Input: dimensioned drawing with shaded views. Units: mm. Origin: part minimum x, y, z. A direction names the side the tool comes from. Round coordinates to 2 decimals unless told otherwise and drop trailing zeros. Loops run counter-clockwise (first coordinate to the right, second up) from the corner with the lowest first, then second, coordinate; pieces in that order, holes last. Notation, with made-up numbers: M -12.75,-12 L 14.25,-12 A21 ccw 14.25,4 Z; hole C 70.5,4.25 d10. An arc over 180 degrees is marked long. Answer as a JSON object with one key per item and string values.
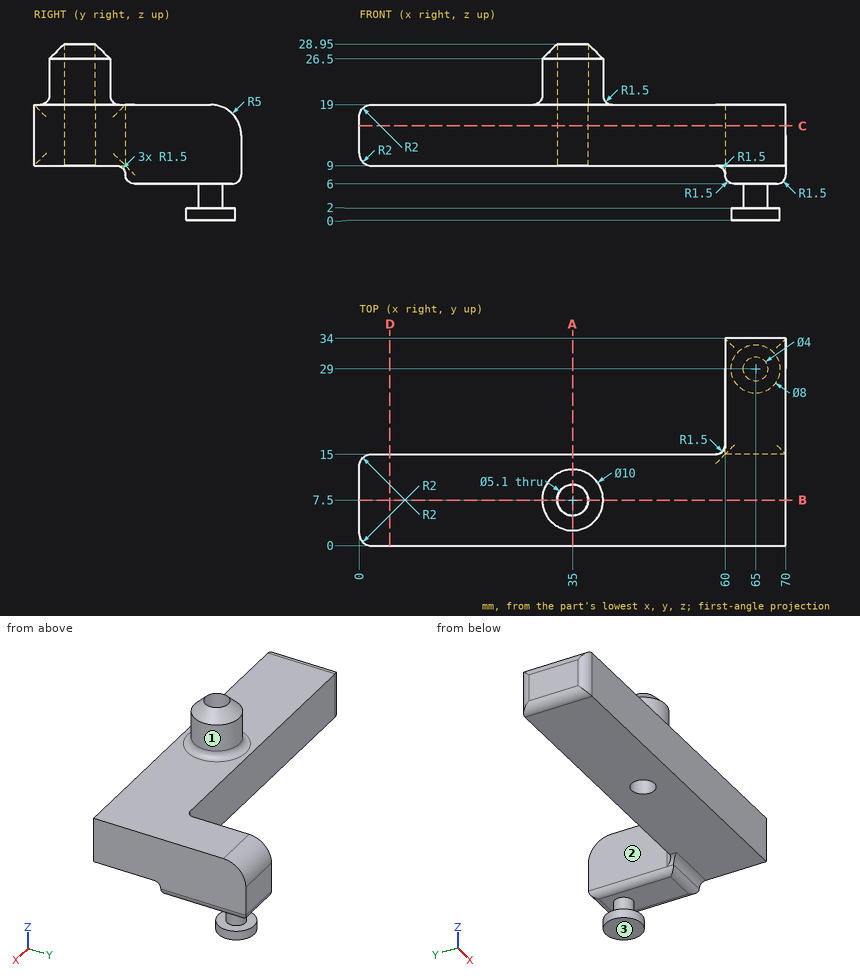
Item 1: Section B-B on y = 7.5. Return the cut outline in (x, z).
Answer sheet:
{"outline": "M 0,11 A2 ccw 2,9 L 32.45,9 L 32.45,28.95 L 30,26.5 L 30,20.5 A1.5 cw 28.5,19 L 2,19 A2 ccw 0,17 Z; M 37.55,9 L 70,9 L 70,19 L 41.5,19 A1.5 cw 40,20.5 L 40,26.5 L 37.55,28.95 Z"}
Item 2: Section C-C on z = 15.5. Return the cut outline in (x, y).
Answer sheet:
{"outline": "M 0,2 A2 ccw 2,0 L 70,0 L 70,33.77 L 60,33.77 L 60,16.5 A1.5 cw 58.5,15 L 2,15 A2 ccw 0,13 Z; hole C 35,7.5 d5.1"}
Item 3: Access query for the marked faces 1, 2 and 3. Directions: +Z, -Z, +X, -X, +Y, -Y. A direction counts if a zero-diameter tool reaches every point of the face in a straight line with its end or side. Return the directions, or none.
Answer sheet:
{"face 1": "+Z", "face 2": "+Z, -Z, -X, +Y", "face 3": "-Z, +X, -X, +Y, -Y"}
Item 4: Section A-A on x = 35. Return the cut outline in (y, z).
Answer sheet:
{"outline": "M 0,9 L 4.95,9 L 4.95,28.95 L 2.5,26.5 L 2.5,20.5 A1.5 cw 1,19 L 0,19 Z; M 10.05,9 L 15,9 L 15,19 L 14,19 A1.5 cw 12.5,20.5 L 12.5,26.5 L 10.05,28.95 Z"}
Item 5: Line query: probe 1 along Y at (x, z) = (35, 16); probe 2 along Y at (x, z) = (35, 24.25); probe 3 along X at (y, z) = (21, 13). Output: solid intervals per line, ascending. Write a range as from..to.
Answer sheet:
{"probe 1": "y = 0..4.95, 10.05..15", "probe 2": "y = 2.5..4.95, 10.05..12.5", "probe 3": "x = 60..70"}
Item 6: Section D-D on x = 5. Return the cut outline in (y, z), then the cut area to 3 significant figures.
Answer sheet:
{"outline": "M 0,9 L 15,9 L 15,19 L 0,19 Z", "area": "150 mm²"}
Item 7: Contact query for flat-ended pins moving along their axis: pin 1 Ø12.5 at (y, z) = (25, 15.5) entering from -X; pin 2 Ø3 at (x, z) = (20.5, 11.5) entering from +Y; pin 3 Ø12 at (x, y) = (32, 4.5) entering from +Z; pin 4 Ø8 at (x, y) = (18.5, 10) entering from -Z. Output: stop coordinate, or through.
Answer sheet:
{"pin 1": "stops at x = 60", "pin 2": "stops at y = 15", "pin 3": "stops at z = 28.95", "pin 4": "stops at z = 9"}
